```python
from build123d import *

# Parameters (mm, degrees)
F1_DEPTH = 1.5875
F3_D     = 4.318
F3_DEPTH = 762
F3_TIP   = 1.2972580765


with BuildPart() as f1:
    # F0 (on Right) → F1 (new body, symmetric)
    with BuildSketch(Plane.YZ):
        Polygon((-101.6, 12.7), (0, 0), (0, 19.05), (-101.6, 19.05), align=None)
    extrude(amount=F1_DEPTH, both=True)

    # F3
    with Locations(Plane.YZ.offset(1.5875)):
        with Locations((-57.15, 11.86942)):
            Hole(F3_D / 2, depth=F3_DEPTH)
            with Locations((0, 0, -(F3_DEPTH + F3_TIP / 2))):  # 118° drill point
                Cone(0, F3_D / 2, F3_TIP, mode=Mode.SUBTRACT)


solid = f1.part
```
Input: part model. Units: mm. Frame: model coordinates. Give positions to 0.01 mm unless a question says otherwise; leave off trailing zeros. Write each loop counter-clockwise with the first axis right and the second up, starting at its lowest first coordinate (ties: lowest second). Pieces come first, ordered by that corner, then holes. Notation, with made-up numbers: (-29.75, 53.25) - (-25.75, 53.25) arc R11 cw to (-25.75, 61.25) - close; hole circle Ø7 at (-3, 66). An arc over 180 degrees is marked (long way). Write item = value, one per line. Start each with the question number.
1) Pin query (flat end, axial travel): pin 1 (1 mm diameter, centred on x = 0.5, y = -50, fed in from -Z). Return the tip coordinate at first contact, or that it passes through.
2) Cut plane A-A (y = -57.15). Return loops of the section in (x, z), and give its area (3 significant figures).
3) Cut plane D-D (z = 7.75). Return loops of the section in (x, y).
4) Cut plane B-B (z = 3.5). Return loops of the section in (x, y).
5) Cut plane C-C (x = 0.8). Return loops of the section in (y, z).
6) Material intervals for L1, parallel to Z at x = -0.25, y = -57.15; L2, parallel to Y at x = -1.05, z = 12.75; L3, parallel to Y at x = 0.55, z = 13.5, sorted ascending. Write a range as [from, to].
7) Draft query along Z for faces 1 (the face through (0, -50, 19.05)), 2 (the face through (-0.02, -56.87, 14.01)), 3 (the face through (0, -101.6, 16)). Return one class per face: pulls with the +Z half, pulls with the -Z half, needs draft (parallel to the pull), parting line crosses it, or undercut.
Answers follow:
q1.pin_1 = 6.19
q2.outline = (-1.59, 7.14) - (1.59, 7.14) - (1.59, 9.71) - (-1.59, 9.71) - close; (-1.59, 14.03) - (1.59, 14.03) - (1.59, 19.05) - (-1.59, 19.05) - close
q2.area = 24.1 mm^2
q3.outline = (-1.59, -62) - (1.59, -62) - (1.59, 0) - (-1.59, 0) - close
q4.outline = (-1.59, -28) - (1.59, -28) - (1.59, 0) - (-1.59, 0) - close
q5.outline = (-101.6, 12.7) - (0, 0) - (0, 19.05) - (-101.6, 19.05) - close; hole circle Ø4.32 at (-57.15, 11.87)
q6.L1 = [7.14, 9.71], [14.03, 19.05]
q6.L2 = [-101.6, -59.12], [-55.18, 0]
q6.L3 = [-101.6, -58.57], [-55.73, 0]
q7.face_1 = pulls with the +Z half
q7.face_2 = undercut
q7.face_3 = needs draft
